Geometry: final body of the model. Coordinates: model frame, mm. A direction names the side the tool comes from. Coordinates: 2 decimals unless noted, no trailing zeros. Write each loop counter-clockwise with the first axis right and the second up, starting at its lowest first coordinate (ties: lowest second). Pieces come first, ordered by that corner, then holes.
from build123d import *

# Parameters (mm, degrees)
SKETCH1_W                = 4
SKETCH1_H                = 5
BOSS_EXTRUDE1_DEPTH      = 3
SKETCH2_W                = 2
SKETCH2_H                = 5
CUT_EXTRUDE1_DEPTH       = 2
BOSS_EXTRUDE2_START      = -1
SKETCH3_R                = 1
BOSS_EXTRUDE2_DEPTH      = 3.5
SKETCH4_W                = 4
SKETCH4_H                = 5.951198117
CUT_EXTRUDE2_DEPTH       = 10.00071436
SKETCH5_W                = 9
SKETCH5_H                = 1
BOSS_EXTRUDE3_DEPTH      = 5
BOSS_EXTRUDE4_DEPTH      = 1.5
BOSS_EXTRUDE4_DEPTH_BACK = 6.5
SKETCH7_W                = 1
SKETCH7_H                = 8
BOSS_EXTRUDE5_DEPTH      = 2


with BuildPart() as part:
    # Sketch1 → Boss-Extrude1 (new body)
    with BuildSketch(Plane.XY):
        Rectangle(SKETCH1_W, SKETCH1_H)
    extrude(amount=BOSS_EXTRUDE1_DEPTH)

    # Sketch2 → Cut-Extrude1 (cut)
    with BuildSketch(Plane.XY.offset(3)):
        Rectangle(SKETCH2_W, SKETCH2_H)
    extrude(amount=-CUT_EXTRUDE1_DEPTH, mode=Mode.SUBTRACT)

    # Sketch3 → Boss-Extrude2 (add)
    with BuildSketch(Plane(origin=(2, 0, 0), x_dir=(0, 0, -1), z_dir=(1, 0, 0)).offset(BOSS_EXTRUDE2_START)):
        with BuildLine():
            Line((0, 2.5), (3, 2.5))
            ThreePointArc((3, 2.5), (5.916707084, 0.416707084), (3.833414169, -2.5))
            Line((3.833414169, -2.5), (0, -2.5))
            Line((0, -2.5), (0, 2.5))
        make_face()
        with Locations((3.416707084, 0)):
            Circle(SKETCH3_R, mode=Mode.SUBTRACT)
    boss_extrude2 = extrude(amount=BOSS_EXTRUDE2_DEPTH)

    # Mirror1: Boss-Extrude2 across plane
    add(boss_extrude2.mirror(Plane(origin=(0, 0, 0), x_dir=(0, 0, 1), z_dir=(1, 0, 0))))

    # Sketch4 → Cut-Extrude2 (cut, through all)
    with BuildSketch(Plane.XZ.offset(2.5)):
        with Locations((0, -2.975599059)):
            Rectangle(SKETCH4_W, SKETCH4_H)
    extrude(amount=-CUT_EXTRUDE2_DEPTH, mode=Mode.SUBTRACT)


with BuildPart() as cut_extrude2_piece_1:
    # of the separate pieces the step leaves, piece 1, a body of its own (cut_extrude2_pieces)
    add(part.part.solids().sort_by_distance((4.5, 2.5, 0))[0])



with BuildPart() as cut_extrude2_piece_2:
    # of the separate pieces the step leaves, piece 2, a body of its own (cut_extrude2_pieces)
    add(part.part.solids().sort_by_distance((-2, 2.5, -3))[0])


with BuildPart() as cut_extrude2_piece_3:
    # of the separate pieces the step leaves, piece 3, a body of its own (cut_extrude2_pieces)
    add(part.part.solids().sort_by_distance((-2, 2.5, 3))[0])


with BuildPart() as cut_extrude2_piece_1_1:
    add(cut_extrude2_piece_1.part)

    add(cut_extrude2_piece_2.part)  # Boss-Extrude3 merges Cut-Extrude2 piece 2

    add(cut_extrude2_piece_3.part)  # Boss-Extrude3 merges Cut-Extrude2 piece 3
    # Sketch5 → Boss-Extrude3 (add)
    with BuildSketch(Plane.XZ.offset(2.5)):
        with Locations((0, 0.5)):
            Rectangle(SKETCH5_W, SKETCH5_H)
    extrude(amount=-BOSS_EXTRUDE3_DEPTH)

    # Sketch6 → Boss-Extrude4 (add, two sides: drawn at the far end of the back side and taken through both)
    with BuildSketch(Plane(origin=(0, 2.5, 0), x_dir=(1, 0, 0), z_dir=(0, 1, 0)).offset(-BOSS_EXTRUDE4_DEPTH_BACK)):
        Polygon((-1, -3), (-1, -1), (1, -1), (1, -3), (2, -3), (2, 0), (-2, 0), (-2, -3), align=None)
    extrude(amount=BOSS_EXTRUDE4_DEPTH + BOSS_EXTRUDE4_DEPTH_BACK)

    # Sketch7 → Boss-Extrude5 (add)
    with BuildSketch(Plane.XY.offset(3)):
        with Locations((1.5, 0)):
            Rectangle(SKETCH7_W, SKETCH7_H)
        with Locations((-1.5, 0)):
            Rectangle(SKETCH7_W, SKETCH7_H)
    extrude(amount=BOSS_EXTRUDE5_DEPTH)


solid = cut_extrude2_piece_1_1.part
Item 1: Section C-C, the plane z = -4. Output: boundary loops of the cut face in (x, y), plus the area to 3 significant figures.
Derived:
outline: (-4.5, -2.47) - (-2, -2.47) - (-2, -0.81) - (-4.5, -0.81) - close; (-4.5, 0.81) - (-2, 0.81) - (-2, 2.47) - (-4.5, 2.47) - close; (2, -2.47) - (4.5, -2.47) - (4.5, -0.81) - (2, -0.81) - close; (2, 0.81) - (4.5, 0.81) - (4.5, 2.47) - (2, 2.47) - close
area: 16.5 mm2
Item 2: Set-up query: faces 4 (the flat face through (3, -2.5, -1)), 5 (the flat face through (-3, -2.5, -1)), 6 (the flat face through (3, 2.5, -1)), 7 (the flat face through (-3, 0, 1)), 8 (the flat face through (-1, 0, 3)). Return all of +Z, -Z, +X, -X, +Y, -Y with unobstructed straight access to the full face (end or side cutting, diameter ignored); none if empty.
Derived:
face 4: +Z, -Z, +X, -Y
face 5: +Z, -Z, -X, -Y
face 6: +Z, +X, +Y
face 7: +Z, -X, +Y, -Y
face 8: +Z, +Y, -Y
Item 3: Section D-D, the plane y = -2.75. Output: boundary loops of the cut face in (x, z), plus the area to 3 significant figures.
Derived:
outline: (-2, 0) - (2, 0) - (2, 5) - (1, 5) - (1, 1) - (-1, 1) - (-1, 5) - (-2, 5) - close
area: 12.0 mm2
Item 4: Section B-B, the plane y = 0. Output: boundary loops of the cut face in (x, z).
Derived:
outline: (-4.5, -5.95) - (-2, -5.95) - (-2, -4.42) - (-4.5, -4.42) - close; (-4.5, -2.42) - (-2, -2.42) - (-2, 0) - (2, 0) - (2, -2.42) - (4.5, -2.42) - (4.5, 1) - (2, 1) - (2, 5) - (1, 5) - (1, 1) - (-1, 1) - (-1, 5) - (-2, 5) - (-2, 1) - (-4.5, 1) - close; (2, -5.95) - (4.5, -5.95) - (4.5, -4.42) - (2, -4.42) - close
Item 5: Section A-A, the plane z = 2.25. Output: boundary loops of the cut face in (x, y).
Derived:
outline: (-2, -4) - (-1, -4) - (-1, 4) - (-2, 4) - close; (1, -4) - (2, -4) - (2, 4) - (1, 4) - close
Item 6: Pin query (flat end, axial travel): pin 1 (2 mm diameter, centred on x = 3.5, y = -1, fed in from +Z); pin 2 (3 mm diameter, centred on x = -3, z = -2, fed in from +Y); pin 3 (1.2 mm diameter, centred on x = 3.5, z = -2, fed in from -Y). Return the tip coordinate at first contact, or that it passes through.
Derived:
pin 1: stops at z = 1
pin 2: stops at y = 2.53
pin 3: stops at y = -2.5
Item 7: Material intervals for probe 1 along X at (y, z) = (0.25, -1.25); probe 2 along X at (y, z) = (3.25, 4.25); probe 3 along Z at (x, y) = (3.4, 0), sorted ascending.
Derived:
probe 1: x = -4.5 to -2, 2 to 4.5
probe 2: x = -2 to -1, 1 to 2
probe 3: z = -5.95 to -4.42, -2.42 to 1
Item 8: Pull-direction query (X, two-part tool) for faces 1 (the flat face through (-3, 2.5, -1)), 2 (the flat face through (-4.5, 0, -2)), 3 (the flat face through (0, 0, 0)); classes: released by +X, released by -X, zero draft, split by the parting line, or undercut.
Derived:
face 1: zero draft
face 2: released by -X
face 3: undercut
